The listing builds one solid part. Answer for the finished solid, in the listing's coordinates (mm). Coordinates: 2 decimals unless noted, no trailing zeros. Loops run counter-clockwise (first coordinate to the right, second up) from the corner with the lowest first, then second, coordinate; pieces in that order, holes last. Notation, with made-up numbers: M 86.5,30.5 L 127.5,30.5 A11 ccw 127.5,43.5 Z; hole C -11,48.5 d2. An arc over 180 degrees is marked long. Return JSON: item names as keys, results as strings. Group by question number.
1. Section B-B (y = 1.9) is taken. Write down the section's boundary in (x, z), then the cut area to 3 significant figures.
2. Section A-A (z = 0.25) is taken. Write down the section's boundary in (x, y), then the cut area to 3 significant figures.
3. Straight lines are drawn through the part: L1, parallel to X at y = 2, z = -4; L2, parallel to Z at x = -6, y = 1.9; L3, parallel to Y at x = -15, z = 9.75. For each, find the intervals that lie inside material, in ascending order. Write a range as from..to.
4. Given P1, Ø0.6, axis at y = 2.5, z = -4, coming from the +X side; P2, Ø3, axis at x = -3.5, y = 0.5, coming from the +Z side; P3, Ø1.6, axis at x = -4, y = 2.5, coming from the -Z side; P4, Ø0.6, axis at y = 2, z = -4.5, coming from the -X side, each flat-ended and moving along its own axis, determine where each tip first touches the part or whether it passes through.
5. Section C-C (x = -12.5) is taken. Write down the section's boundary in (y, z), then the cut area to 3 significant figures.
```python
from build123d import *

# Parameters (mm, degrees)
SKETCH1_W           = 29.8
SKETCH1_H           = 24.8
BOSS_EXTRUDE1_DEPTH = 3
SKETCH2_W           = 32
SKETCH2_H           = 27
BOSS_EXTRUDE2_DEPTH = 2
CHAMFER1_SIZE       = 1


with BuildPart() as part:
    # Sketch1 → Boss-Extrude1 (new body)
    with BuildSketch(Plane(origin=(0, 0, 0), x_dir=(1, 0, 0), z_dir=(0, 1, 0))):
        Rectangle(SKETCH1_W, SKETCH1_H)
    extrude(amount=BOSS_EXTRUDE1_DEPTH)

    # Sketch2 → Boss-Extrude2 (add)
    with BuildSketch(Plane(origin=(0, 3, 0), x_dir=(1, 0, 0), z_dir=(0, 1, 0))):
        Rectangle(SKETCH2_W, SKETCH2_H)
    extrude(amount=BOSS_EXTRUDE2_DEPTH)

    # Chamfer1
    chamfer1_edges = [part.edges().sort_by_distance(p)[0] for p in [
        (0, 0, -12.4),
        (14.9, 0, 0),
        (0, 0, 12.4),
        (-14.9, 0, 0),
        (-14.9, 1.5, -12.4),
        (14.9, 1.5, -12.4),
        (14.9, 1.5, 12.4),
        (-14.9, 1.5, 12.4),
    ]]
    chamfer(chamfer1_edges, length=CHAMFER1_SIZE)


solid = part.part
```
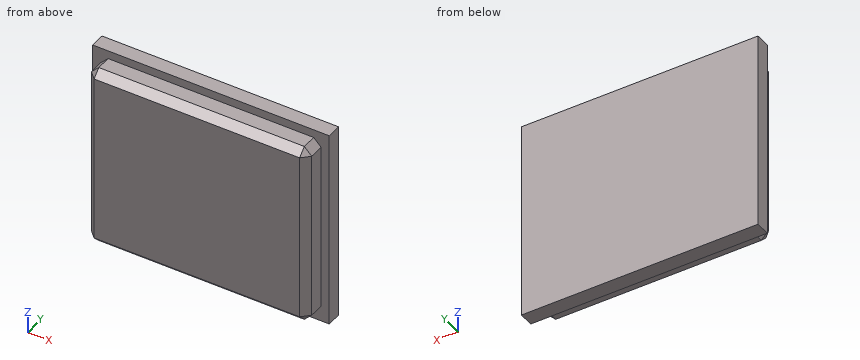
Worked out:
{
 "1": {"outline": "M -14.9,-11.4 L -13.9,-12.4 L 13.9,-12.4 L 14.9,-11.4 L 14.9,11.4 L 13.9,12.4 L -13.9,12.4 L -14.9,11.4 Z", "area": "737 mm^2"},
 "2": {"outline": "M -16,3 L -14.9,3 L -14.9,1 L -13.9,0 L 13.9,0 L 14.9,1 L 14.9,3 L 16,3 L 16,5 L -16,5 Z", "area": "152 mm^2"},
 "3": {"L1": "-14.9..14.9", "L2": "-12.4..12.4", "L3": "3..5"},
 "4": {"P1": "x = 14.9", "P2": "z = 12.4", "P3": "z = -13.5", "P4": "x = -14.9"},
 "5": {"outline": "M 0,-11.4 L 1,-12.4 L 3,-12.4 L 3,-13.5 L 5,-13.5 L 5,13.5 L 3,13.5 L 3,12.4 L 1,12.4 L 0,11.4 Z", "area": "127 mm^2"}
}
